Geometry check sheet. Reference: the model listing, model coordinates, mm. A direction names the side the tool comes from. Give positions to 0.01 mm unless a question says otherwise; leave off trailing zeros. Order: outer loops, then holes, each group sorted by start corner. A loop starts at its lowest first (then second) coordinate and runs counter-clockwise, first axis right, second up. Notation, with made-up numbers: M 17.5,29.25 L 44.5,29.25 A31 ccw 44.5,57.25 Z; hole C 29.25,52 d7. An arc over 180 degrees is marked long. Answer as CSV lines item,"result". Start each with the question number.
```python
from build123d import *

# Parameters (mm, degrees)
SKETCH1_W               = 7.2
SKETCH1_H               = 12
BOSS_EXTRUDE2_DEPTH     = 6
SHELL1_T                = 2
SKETCH4_R               = 1.25
CUT_EXTRUDE2_DEPTH      = 28.897132469
CUT_EXTRUDE2_DEPTH_BACK = 2
SKETCH5_W               = 10
SKETCH5_H               = 16
BOSS_EXTRUDE3_DEPTH     = 4
SHELL2_T                = -3
FILLET1_R               = 1


with BuildPart() as part:
    # Sketch1 → Boss-Extrude2 (new body)
    with BuildSketch(Plane.XY):
        with Locations((19.9, 0)):
            Rectangle(SKETCH1_W, SKETCH1_H)
    extrude(amount=BOSS_EXTRUDE2_DEPTH)

    # Shell1
    shell1_openings = [part.faces().sort_by_distance(p)[0] for p in [
        (16.3, 0, 3),
    ]]
    offset(amount=SHELL1_T, openings=shell1_openings, kind=Kind.INTERSECTION)

    # Sketch4 → Cut-Extrude2 (cut, two sides)
    with BuildSketch(Plane.XY) as cut_extrude2_sk:
        with Locations((20, -3)):
            Circle(SKETCH4_R)
        with Locations((20, 3)):
            Circle(SKETCH4_R)
    extrude(amount=CUT_EXTRUDE2_DEPTH, mode=Mode.SUBTRACT)
    extrude(cut_extrude2_sk.sketch, amount=-CUT_EXTRUDE2_DEPTH_BACK, mode=Mode.SUBTRACT)

    # Sketch5 → Boss-Extrude3 (add)
    with BuildSketch(Plane(origin=(25.5, 0, 0), x_dir=(0, 0, -1), z_dir=(1, 0, 0))):
        with Locations((-3, 0)):
            Rectangle(SKETCH5_W, SKETCH5_H)
    extrude(amount=BOSS_EXTRUDE3_DEPTH)

    # Shell2
    shell2_openings = [part.faces().sort_by_distance(p)[0] for p in [
        (29.5, 0, 3),
    ]]
    offset(amount=SHELL2_T, openings=shell2_openings, kind=Kind.INTERSECTION)

    # Fillet1
    fillet1_edges = [part.edges().sort_by_distance(p)[0] for p in [
        (22.9, -8, 8),
        (22.9, -8, -2),
        (22.9, 8, -2),
        (22.9, 8, 8),
    ]]
    fillet(fillet1_edges, radius=FILLET1_R)


solid = part.part
```
Item 1: Section check B-B on x = 20. Record the boundary of the cut face in (y, z), then the cut area to 3 significant figures.
Item 2: Depth check by flat-ended pin: pin 1 Ø1.5 at (x, y) = (20, 3) entering from +Z. Enter the tip coordinate at first touch or a pass-through.
Item 3: Section check D-D on z = -0.5. Record the boundary of the cut face in (x, y).
Item 4: Draft check along X on faces 1 (the face through (28, -5, 3)), 2 (the face through (21.19, 3.38, 6.99)), 3 (the face through (29.5, 0.1, 5.3)). Enter one of: pulls with the +X half, pulls with the -X half, needs draft (parallel to the pull), parting line crosses it, or undercut.
Item 5: Access from +Z, -Z, +X, -X, +Y, -Y to the whole of each face (thin tool, end or side, straight path). Record for faces 4 (the face through (22.808, 7.699, 7.715)), 5 (the face through (20, 6, 3)), 6 (the face through (28, 0, 1)).
Item 6: Scan lines: line 1 along Y through (x, z) = (20, 6.55); line 2 along Z through (x, y) = (21.5, 4.25); line 3 along X through (y, z) = (-3, 6.55). Record each from-to range of solid material in increasing order.
Item 7: Section check C-C on x = 21.5. Record the boundary of the cut face in (y, z), then the cut area to 3 significant figures.
Item 8: Section check A-A on y = 3. Record the boundary of the cut face in (x, z), then the cut area to 3 significant figures.
Numbers:
1,outline,"M -8,-1 A1 ccw -7,-2 L -4.25,-2 L -4.25,0 L -6,0 L -6,6 L -4.25,6 L -4.25,8 L -7,8 A1 ccw -8,7 Z; M -1.75,-2 L 1.75,-2 L 1.75,0 L -1.75,0 Z; M -1.75,6 L 1.75,6 L 1.75,8 L -1.75,8 Z; M 4.25,-2 L 7,-2 A1 ccw 8,-1 L 8,7 A1 ccw 7,8 L 4.25,8 L 4.25,6 L 6,6 L 6,0 L 4.25,0 Z"
1,area,"67.1 mm2"
2,pin 1,"through"
3,outline,"M 16.3,-8 L 29.5,-8 L 29.5,8 L 16.3,8 Z; hole C 20,-3 d2.5; hole C 20,3 d2.5"
4,face 1,"needs draft"
4,face 2,"undercut"
4,face 3,"pulls with the +X half"
5,face 4,"+Z, +X, -X, +Y"
5,face 5,"-X"
5,face 6,"+X"
6,line 1,"-8 to -4.25, -1.75 to 1.75, 4.25 to 8"
6,line 2,"-2 to 0, 6 to 8"
6,line 3,"16.3 to 18.75, 21.25 to 29.5"
7,outline,"M -8,-1 A1 ccw -7,-2 L 7,-2 A1 ccw 8,-1 L 8,7 A1 ccw 7,8 L -7,8 A1 ccw -8,7 Z; hole M -6,0 L 6,0 L 6,6 L -6,6 Z"
7,area,"87.1 mm2"
8,outline,"M 16.3,-2 L 18.75,-2 L 18.75,0 L 16.3,0 Z; M 16.3,6 L 18.75,6 L 18.75,8 L 16.3,8 Z; M 21.25,-2 L 29.5,-2 L 29.5,1 L 26.5,1 L 26.5,5 L 29.5,5 L 29.5,8 L 21.25,8 L 21.25,6 L 23.5,6 L 23.5,0 L 21.25,0 Z"
8,area,"66.8 mm2"
